Geometry check sheet. Reference: drawing and pictorial views, mm from the part's lowest x, y, z. Give positions to 0.01 mm unless a question says otherwise; leave off trailing zeros. Order: outer loops, then holes, each group sorted by start corner. A loop starts at its lowest first (then second) coordinate and runs counter-clockwise, first axis right, second up. Notation, with made-up numbers: (15.25, -24) - (74.25, -24) arc R22 ccw to (74.25, -14) - close; hole circle Ø6 at (-29.5, 71). An arc over 180 degrees is marked (long way). Answer in a Markdown table with one row per item.
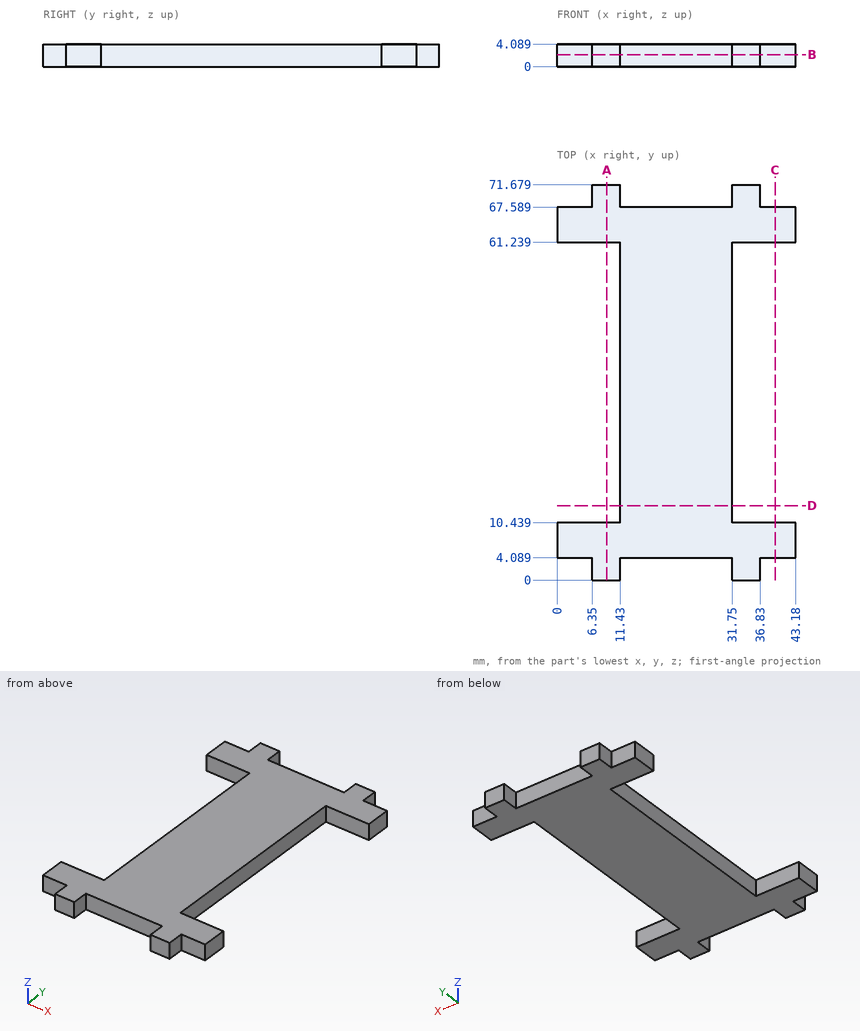
(1) Cross-section at D-D, the plane y = 13.5. Record the cut outline in (x, z).
Geometry says:
| item | result |
|---|---|
| outline | (11.43, 0) - (31.75, 0) - (31.75, 4.09) - (11.43, 4.09) - close |
(2) Gauge pin test, flat ends, axial feed: P1, Ø2, axis at x = 4, z = 2, coming from the -Y side; P2, Ø2, axis at x = 3.5, z = 1.5, coming from the +Y side; P3, Ø1.2, axis at y = 26.5, z = 2.5, coming from the +X side. Record the tip position at first contact, or that the pin passes through.
Geometry says:
| item | result |
|---|---|
| P1 | y = 4.09 |
| P2 | y = 67.59 |
| P3 | x = 31.75 |
(3) Cross-section at A-A, the plane x = 9. Record the cut outline in (y, z).
Geometry says:
| item | result |
|---|---|
| outline | (0, 0) - (10.44, 0) - (10.44, 4.09) - (0, 4.09) - close; (61.24, 0) - (71.68, 0) - (71.68, 4.09) - (61.24, 4.09) - close |
(4) Cross-section at B-B, the plane z = 2.15. Record the cut outline in (x, y).
Geometry says:
| item | result |
|---|---|
| outline | (0, 4.09) - (6.35, 4.09) - (6.35, 0) - (11.43, 0) - (11.43, 4.09) - (31.75, 4.09) - (31.75, 0) - (36.83, 0) - (36.83, 4.09) - (43.18, 4.09) - (43.18, 10.44) - (31.75, 10.44) - (31.75, 61.24) - (43.18, 61.24) - (43.18, 67.59) - (36.83, 67.59) - (36.83, 71.68) - (31.75, 71.68) - (31.75, 67.59) - (11.43, 67.59) - (11.43, 71.68) - (6.35, 71.68) - (6.35, 67.59) - (0, 67.59) - (0, 61.24) - (11.43, 61.24) - (11.43, 10.44) - (0, 10.44) - close |
(5) Thickness scan on L1, parallel to Y at x = 38.5, z = 1.65; L2, parallel to Y at x = 35.5, z = 3.1; L3, parallel to X at y = 68, z = 3.15. Record the ranges inside material, lowest first.
Geometry says:
| item | result |
|---|---|
| L1 | 4.09 to 10.44, 61.24 to 67.59 |
| L2 | 0 to 10.44, 61.24 to 71.68 |
| L3 | 6.35 to 11.43, 31.75 to 36.83 |
(6) Cross-section at C-C, the plane x = 39.5. Record the cut outline in (y, z).
Geometry says:
| item | result |
|---|---|
| outline | (4.09, 0) - (10.44, 0) - (10.44, 4.09) - (4.09, 4.09) - close; (61.24, 0) - (67.59, 0) - (67.59, 4.09) - (61.24, 4.09) - close |
